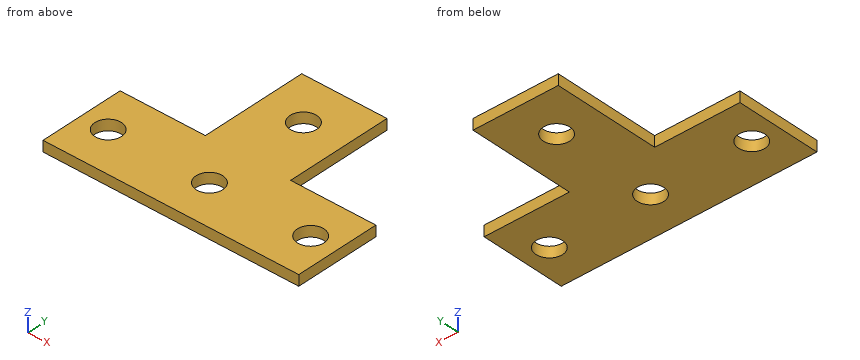
from build123d import *

# Parameters (mm, degrees)
SKETCH2_R           = 2.5
EXTRUDE1_DEPTH      = 2
SKETCH_1_W          = 16
SKETCH_1_H          = 34
CUT_EXTRUDE_1_DEPTH = 60.126981996


with BuildPart() as part:
    # Sketch2 → Extrude1 (new body)
    with BuildSketch(Plane.XY):
        Polygon((-8, 0), (-8, 54), (8, 54), (8, 0), (24, 0), (24, -16), (-24, -16), (-24, 0), align=None)
        with Locations((19, -8)):
            Circle(SKETCH2_R, mode=Mode.SUBTRACT)
        with Locations((0, -8)):
            Circle(SKETCH2_R, mode=Mode.SUBTRACT)
        with Locations((-19, -8)):
            Circle(SKETCH2_R, mode=Mode.SUBTRACT)
        with Locations((0, 43.75)):
            Circle(SKETCH2_R, mode=Mode.SUBTRACT)
        with Locations((0, 11.5)):
            Circle(SKETCH2_R, mode=Mode.SUBTRACT)
    extrude(amount=EXTRUDE1_DEPTH)

    # Эскиз1 → Вырез-Вытянуть1 (cut, through all)
    with BuildSketch(Plane.XY.offset(2)):
        with Locations((0, 37)):
            Rectangle(SKETCH_1_W, SKETCH_1_H)
    extrude(amount=-CUT_EXTRUDE_1_DEPTH, mode=Mode.SUBTRACT)


solid = part.part
Design review of the part built by this model. Coordinates are the model's own, in mm. Coordinates: 2 decimals unless noted, no trailing zeros. Write each loop counter-clockwise with the first axis right and the second up, starting at its lowest first coordinate (ties: lowest second). Pieces come first, ordered by that corner, then holes. Notation, with made-up numbers: (81, -28.75) - (117, -28.75) arc R9 ccw to (117, -21.75) - close; hole circle Ø5 at (43.5, 51.25). An arc over 180 degrees is marked (long way). One line per item, written item: value.
1) Add section A-A (y = 11.5). State the section outline as (x, z) points, plus the area to 3 significant figures.
Answer sheet:
outline: (-8, 0) - (-2.5, 0) - (-2.5, 2) - (-8, 2) - close; (2.5, 0) - (8, 0) - (8, 2) - (2.5, 2) - close
area: 22.0 mm2
2) To check wall thickness, follow probe 1 along Y at (x, z) = (0, 0.85); probe 2 along X at (y, z) = (-7.5, 1.1); probe 3 along Y at (x, z) = (-19, 1.45). State the ranges of each line that lie inside material, in increasing order.
Answer sheet:
probe 1: y = -16 to -10.5, -5.5 to 9, 14 to 20
probe 2: x = -24 to -21.45, -16.55 to -2.45, 2.45 to 16.55, 21.45 to 24
probe 3: y = -16 to -10.5, -5.5 to 0
3) Add section B-B (z = 1.3). State the section outline as (x, y) points.
Answer sheet:
outline: (-24, -16) - (24, -16) - (24, 0) - (8, 0) - (8, 20) - (-8, 20) - (-8, 0) - (-24, 0) - close; hole circle Ø5 at (-19, -8); hole circle Ø5 at (0, -8); hole circle Ø5 at (0, 11.5); hole circle Ø5 at (19, -8)
4) Insertion check: pin 1 (1 mm diameter, centred on x = -15.5, z = 1, fed in from +Y); pin 2 (1 mm diameter, centred on y = 7.5, z = 0.5, fed in from +X); pin 3 (0.6 mm diameter, centred on y = 7.5, z = 1, fed in from -X). Each pin has a flat end and moves straight along its axis. Give the tip position at first contact, or say it passes through.
Answer sheet:
pin 1: stops at y = 0
pin 2: stops at x = 8
pin 3: stops at x = -8
5) Add section D-D (x = 19). State the section outline as (y, z) points, plus the area to 3 significant figures.
Answer sheet:
outline: (-16, 0) - (-10.5, 0) - (-10.5, 2) - (-16, 2) - close; (-5.5, 0) - (0, 0) - (0, 2) - (-5.5, 2) - close
area: 22.0 mm2
6) Add section C-C (x = 0). State the section outline as (y, z) points.
Answer sheet:
outline: (-16, 0) - (-10.5, 0) - (-10.5, 2) - (-16, 2) - close; (-5.5, 0) - (9, 0) - (9, 2) - (-5.5, 2) - close; (14, 0) - (20, 0) - (20, 2) - (14, 2) - close
